from build123d import *

# Parameters (mm, degrees)
F1_DEPTH     = 15
F2_R         = 1.5
F3_T4_DEPTH  = 7.8150729064
F3_T9_DEPTH  = 7.8150729064
F3_T14_DEPTH = 7.8150729064
F3_T19_DEPTH = 7.8150729064
F3_T25_DEPTH = 7.8150729064
F3_T29_DEPTH = 7.8150729064
F3_T36_DEPTH = 7.8150729064
F3_T40_DEPTH = 7.8150729064


# Not quite as in the source:
# - a fillet or chamfer that OpenCascade refuses, or shapes differently, is made with other operations: its cross-section is extruded or revolved along the edge and cut away or added


with BuildPart() as f1:
    # F0 (on Front) → F1 (new body)
    with BuildSketch(Plane.XZ):
        Polygon((0, 5), (0, 0), (2, 0), (6, 3.5), (10, 0), (12, 0), (12, 5), align=None)
    extrude(amount=F1_DEPTH)

    # F2
    f2_edges = [f1.edges().sort_by_distance(p)[0] for p in [
        (0, -15, 2.5),
        (12, -15, 2.5),
        (12, 0, 2.5),
        (0, 0, 2.5),
    ]]
    fillet(f2_edges, radius=F2_R)

    # F3: fillet of radius 0.5 on 4 edges, made by hand


with BuildPart() as f3_tool2:
    # F3_s3 → F3_t4 (new body)
    with BuildSketch(Plane(origin=(0.1920224944, 0, 0.1680196826), x_dir=(0, 1, 0), z_dir=(0.7525766947, 0, 0.6585046079))):
        with BuildLine():
            ThreePointArc((-15, -0.8170092157), (-14.8535533906, -1.1705626063), (-14.5, -1.3170092157))
            Line((-14.5, -1.3170092157), (-15, -1.3170092157))
            Line((-15, -1.3170092157), (-15, -0.8170092157))
        make_face()
    extrude(amount=F3_T4_DEPTH)

    split(bisect_by=Plane(origin=(4.3362831858, 0, 4.9557522124), x_dir=(0, 1, 0), z_dir=(-0.6585046079, 0, -0.7525766947)), keep=Keep.TOP)


with BuildPart() as f1_1:
    add(f1.part)

    # F3_t1: cut F3_tool2
    add(f3_tool2.part, mode=Mode.SUBTRACT)


with BuildPart() as f3_tool7:
    # F3_s8 → F3_t9 (new body)
    with BuildSketch(Plane(origin=(0.7229959458, 0, -0.6326214526), x_dir=(0, 1, 0), z_dir=(0.7525766947, 0, -0.6585046079))):
        with BuildLine():
            ThreePointArc((-15, 7.0850460787), (-14.8535533906, 6.7314926881), (-14.5, 6.5850460787))
            Line((-14.5, 6.5850460787), (-15, 6.5850460787))
            Line((-15, 6.5850460787), (-15, 7.0850460787))
        make_face()
    extrude(amount=F3_T9_DEPTH)

    split(bisect_by=Plane(origin=(0.8672566372, 0, -0.9911504425), x_dir=(0, 1, 0), z_dir=(0.6585046079, 0, -0.7525766947)), keep=Keep.TOP)


with BuildPart() as f1_2:
    add(f1_1.part)

    # F3_t6: cut F3_tool7
    add(f3_tool7.part, mode=Mode.SUBTRACT)


with BuildPart() as f3_tool12:
    # F3_s13 → F3_t14 (new body)
    with BuildSketch(Plane(origin=(0.1920224944, 0, 0.1680196826), x_dir=(0, 1, 0), z_dir=(0.7525766947, 0, 0.6585046079))):
        with BuildLine():
            ThreePointArc((0, -0.8170092157), (-0.1464466094, -1.1705626063), (-0.5, -1.3170092157))
            Line((-0.5, -1.3170092157), (0, -1.3170092157))
            Line((0, -1.3170092157), (0, -0.8170092157))
        make_face()
    extrude(amount=F3_T14_DEPTH)

    split(bisect_by=Plane(origin=(4.3362831858, 0, 4.9557522124), x_dir=(0, 1, 0), z_dir=(-0.6585046079, 0, -0.7525766947)), keep=Keep.TOP)


with BuildPart() as f1_3:
    add(f1_2.part)

    # F3_t11: cut F3_tool12
    add(f3_tool12.part, mode=Mode.SUBTRACT)


with BuildPart() as f3_tool17:
    # F3_s18 → F3_t19 (new body)
    with BuildSketch(Plane(origin=(0.7229959458, 0, -0.6326214526), x_dir=(0, 1, 0), z_dir=(0.7525766947, 0, -0.6585046079))):
        with BuildLine():
            ThreePointArc((0, 7.0850460787), (-0.1464466094, 6.7314926881), (-0.5, 6.5850460787))
            Line((-0.5, 6.5850460787), (0, 6.5850460787))
            Line((0, 6.5850460787), (0, 7.0850460787))
        make_face()
    extrude(amount=F3_T19_DEPTH)

    split(bisect_by=Plane(origin=(0.8672566372, 0, -0.9911504425), x_dir=(0, 1, 0), z_dir=(0.6585046079, 0, -0.7525766947)), keep=Keep.TOP)


with BuildPart() as f1_4:
    add(f1_3.part)

    # F3_t16: cut F3_tool17
    add(f3_tool17.part, mode=Mode.SUBTRACT)


with BuildPart() as f3_tool23:
    # F3_s24 → F3_t25 (new body)
    with BuildSketch(Plane(origin=(0.1920224944, 0, 0.1680196826), x_dir=(0, 1, 0), z_dir=(0.7525766947, 0, 0.6585046079))):
        with BuildLine():
            ThreePointArc((-15, -0.8170092157), (-14.8535533906, -1.1705626063), (-14.5, -1.3170092157))
            Line((-14.5, -1.3170092157), (-15, -1.3170092157))
            Line((-15, -1.3170092157), (-15, -0.8170092157))
        make_face()
    extrude(amount=F3_T25_DEPTH)

    split(bisect_by=Plane(origin=(4.3362831858, 0, 4.9557522124), x_dir=(0, 1, 0), z_dir=(0.6585046079, 0, 0.7525766947)), keep=Keep.TOP)


with BuildPart() as f3_tool27:
    # F3_s28 → F3_t29 (new body)
    with BuildSketch(Plane(origin=(0.7229959458, 0, -0.6326214526), x_dir=(0, 1, 0), z_dir=(0.7525766947, 0, -0.6585046079))):
        with BuildLine():
            ThreePointArc((-15, 7.0850460787), (-14.8535533906, 6.7314926881), (-14.5, 6.5850460787))
            Line((-14.5, 6.5850460787), (-15, 6.5850460787))
            Line((-15, 6.5850460787), (-15, 7.0850460787))
        make_face()
    extrude(amount=F3_T29_DEPTH)

    split(bisect_by=Plane(origin=(0.8672566372, 0, -0.9911504425), x_dir=(0, 1, 0), z_dir=(-0.6585046079, 0, 0.7525766947)), keep=Keep.TOP)


with BuildPart() as f3_tool23_1:
    add(f3_tool23.part)

    # F3_t31: intersect F3_tool27
    add(f3_tool27.part, mode=Mode.INTERSECT)


with BuildPart() as f1_5:
    add(f1_4.part)

    # F3_t21: cut F3_tool23
    add(f3_tool23_1.part, mode=Mode.SUBTRACT)


with BuildPart() as f3_tool34:
    # F3_s35 → F3_t36 (new body)
    with BuildSketch(Plane(origin=(0.1920224944, 0, 0.1680196826), x_dir=(0, 1, 0), z_dir=(0.7525766947, 0, 0.6585046079))):
        with BuildLine():
            ThreePointArc((0, -0.8170092157), (-0.1464466094, -1.1705626063), (-0.5, -1.3170092157))
            Line((-0.5, -1.3170092157), (0, -1.3170092157))
            Line((0, -1.3170092157), (0, -0.8170092157))
        make_face()
    extrude(amount=F3_T36_DEPTH)

    split(bisect_by=Plane(origin=(4.3362831858, 0, 4.9557522124), x_dir=(0, 1, 0), z_dir=(0.6585046079, 0, 0.7525766947)), keep=Keep.TOP)


with BuildPart() as f3_tool38:
    # F3_s39 → F3_t40 (new body)
    with BuildSketch(Plane(origin=(0.7229959458, 0, -0.6326214526), x_dir=(0, 1, 0), z_dir=(0.7525766947, 0, -0.6585046079))):
        with BuildLine():
            ThreePointArc((0, 7.0850460787), (-0.1464466094, 6.7314926881), (-0.5, 6.5850460787))
            Line((-0.5, 6.5850460787), (0, 6.5850460787))
            Line((0, 6.5850460787), (0, 7.0850460787))
        make_face()
    extrude(amount=F3_T40_DEPTH)

    split(bisect_by=Plane(origin=(0.8672566372, 0, -0.9911504425), x_dir=(0, 1, 0), z_dir=(-0.6585046079, 0, 0.7525766947)), keep=Keep.TOP)


with BuildPart() as f3_tool34_1:
    add(f3_tool34.part)

    # F3_t42: intersect F3_tool38
    add(f3_tool38.part, mode=Mode.INTERSECT)


with BuildPart() as f1_6:
    add(f1_5.part)

    # F3_t32: cut F3_tool34
    add(f3_tool34_1.part, mode=Mode.SUBTRACT)


solid = f1_6.part
Could you check a few things on this model? Use its own coordinates, in mm. A direction names the side the tool comes from. Round coordinates to 2 decimals unless told otherwise and drop trailing zeros. Order: outer loops, then holes, each group sorted by start corner. A loop starts at its lowest first (then second) coordinate and runs counter-clockwise, first axis right, second up.
Q1. Please list where these lines run through material, in increasing order: probe 1 along X at (y, z) = (-3.5, 0.2); probe 2 along X at (y, z) = (-12.5, 2.3); probe 3 along Z at (x, y) = (2.5, -12.5).
Geometry says:
probe 1: x = 0 to 2.23, 9.77 to 12
probe 2: x = 0 to 4.63, 7.37 to 12
probe 3: z = 0.44 to 5
Q2. Imagine slicing it at B-B, the plane y = -1.25. List the corners of the cut face in (x, z) for me, then the cut area to 3 significant figures.
Geometry says:
outline: (0.02, 0) - (2, 0) - (6, 3.5) - (10, 0) - (11.98, 0) - (11.98, 5) - (0.02, 5) - close
area: 45.8 mm2
Q3. Imagine slicing it at A-A, the plane y = -8. List the corners of the cut face in (x, z) for me, then the cut area to 3 significant figures.
Geometry says:
outline: (0, 0) - (2, 0) - (6, 3.5) - (10, 0) - (12, 0) - (12, 5) - (0, 5) - close
area: 46.0 mm2
Q4. Thinking about a two-plate mould opening in X: for faces 1 (the face through (8.08, -14.86, 1.88)), 2 (the face through (0, -7, 3)), 3 (the face through (12, -7, 2)), 4 (the face through (6, -7, 5)), which applies, released by +X, released by -X, zero draft, split by the parting line, or undercut?
Geometry says:
face 1: undercut
face 2: released by -X
face 3: released by +X
face 4: zero draft
Q5. I'm going to push flat-ended pins straight in: P1, Ø4, axis at x = 5, y = -11, coming from the -Z side (3 decimals); P2, Ø3, axis at x = 6.5, y = -11.5, coming from the -Z side. Where does each tip first touch, or does it pass through?
Geometry says:
P1: stops at z = 0.875
P2: stops at z = 1.75
Q6. Which directions (+Z, -Z, +X, -X, +Y, -Y) give clear straight access to the entire face, cutting with the end or side of a thin tool? Please do faces 5 (the face through (3.972, -7.402, 1.726)), 6 (the face through (3.85, -14.86, 1.82)), 7 (the face through (3.85, -0.14, 1.82)).
Geometry says:
face 5: -Z, +Y, -Y
face 6: -Z, -Y
face 7: -Z, +Y
